from build123d import *

# Parameters (mm, degrees)
PAD006_DEPTH    = 20
SKETCH009_W     = 12.4
SKETCH009_H     = 4
SKETCH009_H_2   = 2.2
SKETCH009_H_3   = 10.9
PAD007_DEPTH    = 10.2
POCKET002_DEPTH = 19.101
PAD008_START    = -8
PAD008_DEPTH    = 3.4
POCKET003_DEPTH = 2
SKETCH013_R     = 1.4
POCKET004_DEPTH = 1.401
SKETCH015_W     = 2.8
SKETCH015_H     = 4.2
POCKET005_DEPTH = 16


with BuildPart() as part:
    # Sketch008 → Pad006 (new body)
    with BuildSketch(Plane.XZ):
        with BuildLine():
            Line((6.4, 5), (6, 5))
            Line((6, -4.2), (6, 5))
            ThreePointArc((5, -5.2), (5.707107, -4.907107), (6, -4.2))
            Line((-5, -5.2), (5, -5.2))
            ThreePointArc((-6, -4.2), (-5.707107, -4.907107), (-5, -5.2))
            Line((-6, 5), (-6, -4.2))
            Line((-6, 5), (-6.4, 5))
            ThreePointArc((-6.4, 5), (-7.107107, 4.707107), (-7.4, 4))
            Line((-7.4, 4), (-7.4, -5.4))
            ThreePointArc((-7.4, -5.4), (-7.107107, -6.107107), (-6.4, -6.4))
            Line((-6.4, -6.4), (6.4, -6.4))
            ThreePointArc((6.4, -6.4), (7.107107, -6.107107), (7.4, -5.4))
            Line((7.4, -5.4), (7.4, 4))
            ThreePointArc((7.4, 4), (7.107107, 4.707107), (6.4, 5))
        make_face()
    extrude(amount=PAD006_DEPTH)

    # Sketch009 (on Face12 of Pad006) → Pad007 (join)
    with BuildSketch(Plane(origin=(0, 0, -5.2), x_dir=(-1, 0, 0), z_dir=(0, 0, 1))):
        with Locations((0, 2.9)):
            Rectangle(SKETCH009_W, SKETCH009_H)
        with Locations((0, 7)):
            Rectangle(SKETCH009_W, SKETCH009_H_2)
        with Locations((0, 14.55)):
            Rectangle(SKETCH009_W, SKETCH009_H_3)
    extrude(amount=PAD007_DEPTH)

    # Sketch010 (on Face14 of Pad007) → Pocket002 (cut, through all)
    with BuildSketch(Plane(origin=(0, -0.9, 0), x_dir=(1, 0, 0), z_dir=(0, 1, 0))):
        with BuildLine():
            Line((-4, -7.8), (4, -7.8))
            ThreePointArc((4, -7.8), (5.414214, -7.214214), (6, -5.8))
            Line((6, -5.8), (6, 3.2))
            ThreePointArc((6, 3.2), (5.414214, 4.614214), (4, 5.2))
            Line((4, 5.2), (-4, 5.2))
            ThreePointArc((-4, 5.2), (-5.414214, 4.614214), (-6, 3.2))
            Line((-6, 3.2), (-6, -5.8))
            ThreePointArc((-6, -5.8), (-5.414214, -7.214214), (-4, -7.8))
        make_face()
    extrude(amount=-POCKET002_DEPTH, mode=Mode.SUBTRACT)

    # Sketch011 (on Face6 of Pocket002) → Pad008 (join)
    with BuildSketch(Plane(origin=(0, 0, -6.4), x_dir=(1, 0, 0), z_dir=(0, 0, -1)).offset(PAD008_START)):
        with BuildLine():
            Line((-6, 20), (-10, 20))
            ThreePointArc((-10, 20), (-14, 16), (-10, 12))
            Line((-6, 12), (-10, 12))
            Line((-6, 20), (-6, 12))
        make_face()
        with BuildLine():
            Line((6, 20), (10, 20))
            ThreePointArc((10, 12), (14, 16), (10, 20))
            Line((6, 12), (10, 12))
            Line((6, 20), (6, 12))
        make_face()
    extrude(amount=-PAD008_DEPTH)

    # Sketch012 (on Face15 of Pad008) → Pocket003 (cut)
    with BuildSketch(Plane(origin=(0, 0, 1.6), x_dir=(1, 0, 0), z_dir=(0, 0, -1))):
        Polygon((-6.401924, 14.5), (-6.401924, 17.5), (-9, 19), (-11.598076, 17.5), (-11.598076, 14.5), (-9, 13), align=None)
        Polygon((11.598076, 14.5), (11.598076, 17.5), (9, 19), (6.401924, 17.5), (6.401924, 14.5), (9, 13), align=None)
    extrude(amount=-POCKET003_DEPTH, mode=Mode.SUBTRACT)

    # Sketch013 (on Face57 of Pocket003) → Pocket004 (cut, through all)
    with BuildSketch(Plane(origin=(0, 0, 3.6), x_dir=(1, 0, 0), z_dir=(0, 0, -1))):
        with Locations((-9, 16)):
            Circle(SKETCH013_R)
        with Locations((9, 16)):
            Circle(SKETCH013_R)
    extrude(amount=-POCKET004_DEPTH, mode=Mode.SUBTRACT)

    # Sketch015 (on Face8 of Pocket004) → Pocket005 (cut)
    with BuildSketch(Plane(origin=(7.4, 0, 0), x_dir=(0, 0, 1), z_dir=(1, 0, 0))):
        with Locations((2.2, 16)):
            Rectangle(SKETCH015_W, SKETCH015_H)
    extrude(amount=-POCKET005_DEPTH, mode=Mode.SUBTRACT)


with BuildPart() as part_1:
    # Body002 placement: moved
    add(part.part.moved(Location((0, 59, 0))))


solid = part_1.part
Work out the finished part from the listing and answer in its coordinate system (mm). A direction names the side the tool comes from. Give positions to 0.01 mm unless a question says otherwise; leave off trailing zeros. Loops run counter-clockwise (first coordinate to the right, second up) from the corner with the lowest first, then second, coordinate; pieces in that order, holes last. Notation, with made-up numbers: (63, 6.5) -> (107, 6.5) arc R23 cw to (107, 17.5) -> close; hole circle Ø4 at (-33.75, -30). An arc over 180 degrees is marked (long way). Use a Markdown table: item, result. Add a question column.
1. Section C-C on x = 8 is taken. Determine the outline of the cut face in (y, z).
2. Section D-D on z = 4.5 is taken. Determine the outline of the cut face in (x, y), and give its area (3 significant figures).
3. For faces 1 (the cylindrical face through (-7.099, 53.084, 4.715)), 2 (the cylindrical face through (-5.715, 53.607, -4.899)), 3 (the cylindrical face through (7.115, 53.084, 4.699)), 4 (the flat face through (7.6, 43.7, 3.6)), 5 (the flat face through (11.598, 43, 3)), determine the directions among +Z, -Z, +X, -X, +Y, -Y from which every point of the face is accessible in a straight line to the end or side of a thin tool.
4. Determine the mould class of faces 6 (the flat face through (-8.231, 45.556, 2.586)), 7 (the cylindrical face through (5.43, 44.53, -4.6)), 8 (the flat face through (-5.44, 58.1, -4.8)) for opening direction Y: released by +Y, released by -Y, zero draft, split by the parting line, or undercut.
5. Find the intervals of material crossed by probe 1 along X at (y, z) = (43, 3.9); probe 2 along X at (y, z) = (54.75, 2.5); probe 3 along Y at (x, z) = (-9, 4), in increasing order.
6. Section B-B on y = 43 is taken. State how many separate pieces and enclosed holes the cut face has, and give its area (3 significant figures).
7. Flat-ended cylindrical pins translate along their axes: pin 1 Ø12 at (x, y) = (-6.5, 50.5) entering from +Z; pin 2 Ø4 at (y, z) = (43.5, -4) entering from -X; pin 3 Ø3 at (x, y) = (-8.5, 42) entering from -Z; pin 4 Ø0.6 at (y, z) = (42.5, 2.5) entering from +X (3 decimals). Find the tip coordinate at first contact, or state that the pin passes through.
Results below:
| question | item | result |
|---|---|---|
| 1 | outline | (39, 1.6) -> (40.58, 1.6) -> (40.58, 3.6) -> (42.02, 3.6) -> (42.02, 5) -> (39, 5) -> close; (43.98, 3.6) -> (45.42, 3.6) -> (45.42, 1.6) -> (47, 1.6) -> (47, 5) -> (43.98, 5) -> close |
| 2 | outline | (-10, 39) -> (-6, 39) -> (-6, 59) -> (-7.27, 59) -> (-7.27, 47) -> (-10, 47) arc R4 ccw to start; (6, 39) -> (10, 39) arc R4 ccw to (10, 47) -> (7.27, 47) -> (7.27, 59) -> (6, 59) -> close; hole circle Ø2.8 at (-9, 43); hole circle Ø2.8 at (9, 43) |
| 2 | area | 132 mm^2 |
| 3 | face 1 | +Z, -X, +Y |
| 3 | face 2 | +Z |
| 3 | face 3 | +Z, +X, +Y |
| 3 | face 4 | none |
| 3 | face 5 | -Z |
| 4 | face 6 | undercut |
| 4 | face 7 | zero draft |
| 4 | face 8 | released by +Y |
| 5 | probe 1 | x = -14 to -10.4, -7.6 to -6, 6 to 7.6, 10.4 to 14 |
| 5 | probe 2 | x = -7.4 to -6, 6 to 7.4 |
| 5 | probe 3 | y = 39 to 41.6, 44.4 to 47 |
| 6 | separate pieces | 5 |
| 6 | enclosed holes | 0 |
| 6 | area | 60.0 mm^2 |
| 7 | pin 1 | stops at z = 5 |
| 7 | pin 2 | stops at x = -7.4 |
| 7 | pin 3 | stops at z = -6.2 |
| 7 | pin 4 | stops at x = 13.995 |
